For this review, take the finished solid that the model builds, in its own axes (mm). A direction names the side the tool comes from. Round coordinates to 2 decimals unless told otherwise and drop trailing zeros. Write each loop counter-clockwise with the first axis right and the second up, starting at its lowest first coordinate (ties: lowest second). Pieces come first, ordered by that corner, then holes. Notation, with made-up numbers: M 80,24.25 L 113,24.25 A22 cw 113,56.25 Z; hole C 21.5,-7 d5. An arc over 180 degrees is marked long. Use one line per item in the form item = value. Start each with the question number.
Item 1: For line 1 (Z direction, x = -36.25, y = 0); line 2 (Z direction, x = -5.25, y = 0) (3 decimals), list the stretches that pass through material, from the lowest coordinate up. Write a range as [from, to].
Item 2: Draft analysis for pull direction Y (two halves, no side actions). For faces 4 (the flat face through (-12, 2, 18)), 5 (the cylindrical face through (-13.311, -2.737, 12.325)), 6 (the conical face through (-12.31, -4.4, 19.83)), state which applies: released by +Y, released by -Y, zero draft, split by the parting line, or undercut.
Item 3: For P1, Ø3, axis at x = -25.5, y = -16.5, coming from the +Z side; P2, Ø10, axis at x = -6, y = 12, coming from the +Z side; P3, Ø5, axis at x = -26.5, z = -16, coming from the +Y side; P4, Ø12.5, axis at y = 0, z = 0, coming from the -X side (3 decimals), all flat-tipped, find the tip position at first contact; note any pin that passes through.
Item 4: Add section A-A (x = -16). State the section outline as (y, z) points (3 decimals), and give its area (3 significant figures).
Item 5: Add section B-B (x = -43). State the section outline as (y, z) points.
Item 6: For faces 1 (the cylindrical face through (-44.138, -4.336, 19.524)), 2 (the cylindrical face through (-44.916, 6.466, 2.681)), 3 (the cylindrical face through (-6.078, 9.139, -14.334)), list the 3-axis set-ups (+Z, -Z, +X, -X, +Y, -Y) from which the entire face can be reached by the end or side of a thin tool; tool diameter is ignored.
from build123d import *


with BuildPart() as part:
    # Sketch1 → Base-Revolve (revolve)
    with BuildSketch(Plane.XY):
        with BuildLine():
            Line((0, 12.625), (0, 16.6))
            ThreePointArc((0, 16.6), (-0.117157288, 16.882842712), (-0.4, 17))
            Line((-0.4, 17), (-11.6, 17))
            ThreePointArc((-11.6, 17), (-11.882842712, 17.117157288), (-12, 17.4))
            Line((-12, 17.4), (-12, 20))
            Line((-12, 20), (-17, 25))
            Line((-17, 25), (-31, 25))
            Line((-31, 25), (-33.771281292, 20.2))
            ThreePointArc((-33.771281292, 20.2), (-33.917691454, 20.053589838), (-34.117691454, 20))
            Line((-34.117691454, 20), (-53.882308546, 20))
            ThreePointArc((-53.882308546, 20), (-54.082308546, 20.053589838), (-54.228718708, 20.2))
            Line((-54.228718708, 20.2), (-57, 25))
            Line((-57, 25), (-59, 25))
            ThreePointArc((-59, 25), (-59.707106781, 24.707106781), (-60, 24))
            Line((-60, 24), (-60, 7))
            Line((-60, 7), (-30.247595264, 7))
            Line((-30.247595264, 7), (-27, 12.625))
            Line((-27, 12.625), (0, 12.625))
        make_face()
    revolve(axis=Axis((0, 0, 0), (-1, 0, 0)))


solid = part.part
Calculated:
q1.line_1 = [-20, -7], [7, 20]
q1.line_2 = [-17, -12.625], [12.625, 17]
q2.face_4 = zero draft
q2.face_5 = undercut
q2.face_6 = split by the parting line
q3.P1 = 20
q3.P2 = 15.49
q3.P3 = 21.04
q3.P4 = through
q4.outline = C 0,0 d48; hole C 0,0 d25.25
q4.area = 1,310 mm^2
q5.outline = C 0,0 d40; hole C 0,0 d14
q6.face_1 = none
q6.face_2 = +X, -X
q6.face_3 = +X
